```python
from build123d import *

# Parameters (mm, degrees)
F0_W     = 63.5
F0_H     = 40.64
F0_W_2   = 57.15
F0_H_2   = 34.29
F1_DEPTH = 3.175
F2_DEPTH = 19.05
F3_W     = 57.15
F3_H     = 34.29
F4_DEPTH = 3.175
F5_DEPTH = 19.05


# Not quite as in the source:
# - a length typed as a fraction of an inch, garbled in the dataset ("3 / 203.2 mm" for 3/8 in), is restored


with BuildPart() as f1:
    # F0 (on Top) → F1 (new body)
    with BuildSketch(Plane.XY):
        with Locations((73.5778744221, 64.3721897411)):
            Rectangle(F0_W, F0_H)
        with Locations((73.5778744221, 64.3721897411)):
            Rectangle(F0_W_2, F0_H_2, mode=Mode.SUBTRACT)
        with Locations((73.5778744221, 64.3721897411)):
            Rectangle(F0_W_2, F0_H_2)
    extrude(amount=-F1_DEPTH)

    # F0 (on Top) → F2 (join)
    with BuildSketch(Plane.XY):
        with Locations((73.5778744221, 64.3721897411)):
            Rectangle(F0_W, F0_H)
        with Locations((73.5778744221, 64.3721897411)):
            Rectangle(F0_W_2, F0_H_2, mode=Mode.SUBTRACT)
    extrude(amount=F2_DEPTH)

    # F3 (on face) → F4 (join)
    with BuildSketch(Plane.XY.offset(19.05)):
        Polygon((25.6539992988, 109.8956785083), (25.6539992988, 18.4556785083), (51.0539992988, 18.4556785083), (51.0539992988, 21.6306785083), (28.8289992988, 21.6306785083), (28.8289992988, 106.7206785083), (118.9989992988, 106.7206785083), (118.9989992988, 21.6306785083), (63.7539992988, 21.6306785083), (63.7539992988, 18.4556785083), (122.1739992988, 18.4556785083), (122.1739992988, 109.8956785083), align=None)
        Polygon((51.0539992988, 21.6306785083), (51.0539992988, 18.4556785083), (63.7539992988, 18.4556785083), (63.7539992988, 21.6306785083), (118.9989992988, 21.6306785083), (118.9989992988, 106.7206785083), (28.8289992988, 106.7206785083), (28.8289992988, 21.6306785083), align=None)
        with Locations((73.5778744221, 64.3721897411)):
            Rectangle(F3_W, F3_H, mode=Mode.SUBTRACT)
    extrude(amount=F4_DEPTH)

    # F3 (on face) → F5 (join)
    with BuildSketch(Plane.XY.offset(19.05)):
        Polygon((25.6539992988, 109.8956785083), (25.6539992988, 18.4556785083), (51.0539992988, 18.4556785083), (51.0539992988, 21.6306785083), (28.8289992988, 21.6306785083), (28.8289992988, 106.7206785083), (118.9989992988, 106.7206785083), (118.9989992988, 21.6306785083), (63.7539992988, 21.6306785083), (63.7539992988, 18.4556785083), (122.1739992988, 18.4556785083), (122.1739992988, 109.8956785083), align=None)
    extrude(amount=F5_DEPTH)


solid = f1.part
```
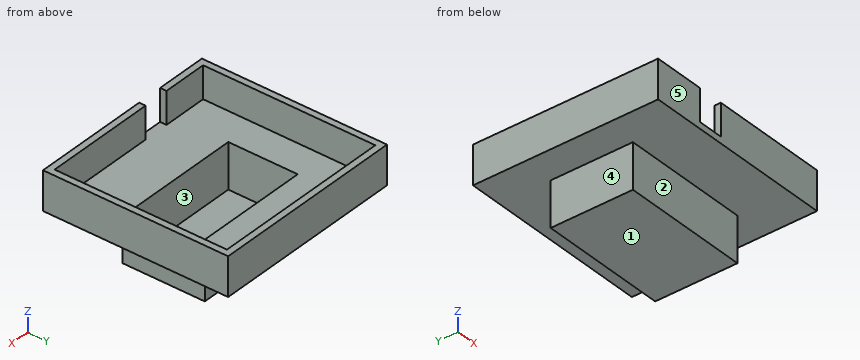
Check sheet for the modelled part. Datum: model origin and axes. Units: mm. Face numbers are marked on the shaded views. A direction names the side the tool comes from. Round coordinates to 2 decimals unless told otherwise and drop trailing zeros. Loops run counter-clockwise (first coordinate to the right, second up) from the corner with the lowest first, then second, coordinate; pieces in that order, holes last. Notation, with made-up numbers: (18.5, 20) -> (47.5, 20) arc R27 cw to (47.5, 52) -> close; hole circle Ø10 at (-30.75, 45.25). An arc over 180 degrees is marked (long way). Write item = value, one per line. Start each with the question number.
1) Thickness scan on probe 1 along X at (y, z) = (33, 36); probe 2 along Y at (x, z) = (86, 28.5); probe 3 along Y at (x, z) = (84, 19.5). Record the ranges inside material, lowest first.
2) Sectioned sample at B-B, the plane x = 60.5. Record the cut outline in (y, z) (3 decimals), plus the area to 3 significant figures.
3) Sectioned sample at A-A, the plane z = 13.5. Record the cut outline in (x, y).
4) Set-up check for the marked faces 1, 2, 3, 4 and 5: record each of +Z, -Z, +X, -X, +Y, -Y from which the full face is reachable in a straight line by a thin tool's end or side.
5) Gauge pin test, flat ends, axial feed: pin 1 Ø6.5 at (x, z) = (60.5, 8.5) entering from -Y; pin 2 Ø6.5 at (y, z) = (59.5, 3) entering from -X; pin 3 Ø6 at (x, y) = (90.5, 61.5) entering from +Z. Record the tip position at first contact, or that the pin passes through.
6) Sectioned sample at D-D, the plane x = 73. Record the cut outline in (y, z) (3 decimals).
7) Sectioned sample at C-C, the plane y = 31. Record the cut outline in (x, z) (3 decimals), plus the area to 3 significant figures.
Results are:
q1.probe_1 = 25.65 to 28.83, 119 to 122.17
q1.probe_2 = 18.46 to 21.63, 106.72 to 109.9
q1.probe_3 = 18.46 to 47.23, 81.52 to 109.9
q2.outline = (18.456, 19.05) -> (44.052, 19.05) -> (44.052, -3.175) -> (84.692, -3.175) -> (84.692, 19.05) -> (109.896, 19.05) -> (109.896, 38.1) -> (106.721, 38.1) -> (106.721, 22.225) -> (81.517, 22.225) -> (81.517, 0) -> (47.227, 0) -> (47.227, 22.225) -> (18.456, 22.225) -> close
q2.area = 482 mm^2
q3.outline = (41.83, 44.05) -> (105.33, 44.05) -> (105.33, 84.69) -> (41.83, 84.69) -> close; hole (45, 47.23) -> (102.15, 47.23) -> (102.15, 81.52) -> (45, 81.52) -> close
q4.face_1 = -Z, +X, -X, +Y, -Y
q4.face_2 = -Z, +X, -X, -Y
q4.face_3 = +Z
q4.face_4 = -Z, -X, +Y, -Y
q4.face_5 = +Z, -Z, +X, -X, -Y
q5.pin_1 = 44.05
q5.pin_2 = 41.83
q5.pin_3 = 0
q6.outline = (18.456, 19.05) -> (44.052, 19.05) -> (44.052, -3.175) -> (84.692, -3.175) -> (84.692, 19.05) -> (109.896, 19.05) -> (109.896, 38.1) -> (106.721, 38.1) -> (106.721, 22.225) -> (81.517, 22.225) -> (81.517, 0) -> (47.227, 0) -> (47.227, 22.225) -> (21.631, 22.225) -> (21.631, 38.1) -> (18.456, 38.1) -> close
q7.outline = (25.654, 19.05) -> (122.174, 19.05) -> (122.174, 38.1) -> (118.999, 38.1) -> (118.999, 22.225) -> (28.829, 22.225) -> (28.829, 38.1) -> (25.654, 38.1) -> close
q7.area = 407 mm^2
